Source: CAD feature listing. Evaluate the final solid. Frame: model axes, mm. A direction names the side the tool comes from. Give positions to 0.01 mm unless a question says otherwise; leave off trailing zeros. Order: outer loops, then holes, each group sorted by start corner. A loop starts at its lowest first (then second) coordinate and runs counter-clockwise, first axis right, second up.
from build123d import *

# Parameters (mm, degrees)
BOSS_EXTRUDE1_DEPTH = 120
BOSS_EXTRUDE2_DEPTH = 120
SKETCH4_W           = 0.8
SKETCH4_H           = 47.4
BOSS_EXTRUDE3_DEPTH = 120
BOSS_EXTRUDE4_DEPTH = 6
SKETCH6_W           = 3.197214061
SKETCH6_H           = 10
SKETCH6_W_2         = 2.544721395
CUT_EXTRUDE1_DEPTH  = 90
SKETCH7_W           = 91.376615624
SKETCH7_H           = 120.194280457
CUT_EXTRUDE3_DEPTH  = 258
SKETCH8_W           = 8
SKETCH8_H           = 30.385133663
CUT_EXTRUDE4_DEPTH  = 4
SKETCH9_R           = 1.35
CUT_EXTRUDE5_DEPTH  = 11
SKETCH10_W          = 29
SKETCH10_H          = 3.5
CUT_EXTRUDE6_DEPTH  = 10
SKETCH11_W          = 115.146040633
SKETCH11_H          = 26.021704098
CUT_EXTRUDE7_DEPTH  = 103
SKETCH12_W          = 27.624810525
SKETCH12_H          = 10
CUT_EXTRUDE8_DEPTH  = 2.5
SKETCH13_R          = 1.35
CUT_EXTRUDE9_DEPTH  = 5


with BuildPart() as part:
    # Sketch1 → Boss-Extrude1 (new body)
    with BuildSketch(Plane(origin=(0, 0, 0), x_dir=(1, 0, 0), z_dir=(0, 1, 0))):
        with BuildLine():
            Line((-55.813088795, 29.403372847), (-55.813088795, -22.596627153))
            ThreePointArc((-55.813088795, -22.596627153), (-52.766075655, -30.195969229), (-45.313088795, -33.585257641))
            Line((-45.313088795, -33.585257641), (-45.313088795, -31.296627153))
            ThreePointArc((-45.313088795, -31.296627153), (-50.969943044, -28.953481402), (-53.313088795, -23.296627153))
            Line((-53.313088795, -23.296627153), (-53.313088795, 30.103372847))
            ThreePointArc((-53.313088795, 30.103372847), (-50.969943044, 35.760227097), (-45.313088795, 38.103372847))
            Line((-45.313088795, 38.103372847), (-45.313088795, 40.392003335))
            ThreePointArc((-45.313088795, 40.392003335), (-52.766075655, 37.002714924), (-55.813088795, 29.403372847))
        make_face()
        with BuildLine():
            Line((-45.313088795, -31.296627153), (-45.313088795, -33.585257641))
            ThreePointArc((-45.313088795, -33.585257641), (-45.063153419, -33.593784407), (-44.813088795, -33.596627153))
            Line((-44.813088795, -33.596627153), (7.186911205, -33.596627153))
            ThreePointArc((7.186911205, -33.596627153), (14.965085798, -30.374801746), (18.186911205, -22.596627153))
            Line((18.186911205, -22.596627153), (18.186911205, 29.403372847))
            ThreePointArc((18.186911205, 29.403372847), (14.965085798, 37.18154744), (7.186911205, 40.403372847))
            Line((7.186911205, 40.403372847), (-45.313088795, 40.403372847))
            Line((-45.313088795, 40.403372847), (-45.313088795, 40.392003335))
            Line((-45.313088795, 40.392003335), (-45.313088795, 38.103372847))
            Line((-45.313088795, 38.103372847), (7.686911205, 38.103372847))
            ThreePointArc((7.686911205, 38.103372847), (13.343765455, 35.760227097), (15.686911205, 30.103372847))
            Line((15.686911205, 30.103372847), (15.686911205, -23.296627153))
            ThreePointArc((15.686911205, -23.296627153), (13.343765455, -28.953481402), (7.686911205, -31.296627153))
            Line((7.686911205, -31.296627153), (-45.313088795, -31.296627153))
        make_face()
    extrude(amount=BOSS_EXTRUDE1_DEPTH)

    # Sketch3 → Boss-Extrude2 (add)
    with BuildSketch(Plane.XZ):
        Polygon((-49.013088795, 31.972735522), (-49.013088795, -37.623215713), (-53.336517426, -34.913867104), (-55.11106611, -29.984565206), (-55.11106611, -26.811210851), (-55.11106611, 25.452378342), (-53.652842224, 27.779331351), (-52.073193111, 30.226675048), align=None)
        Polygon((11.386911205, 31.972735522), (11.386911205, -38.487790626), (13.269736219, -37.809973621), (16.737085445, -32.276969537), (16.568342629, -31.170966754), (16.568342629, 24.789777041), (15.03852436, 28.997230807), align=None)
    extrude(amount=-BOSS_EXTRUDE2_DEPTH)

    # Sketch4 → Boss-Extrude3 (add)
    with BuildSketch(Plane.XZ):
        with Locations((10.986911205, -3.403372847)):
            Rectangle(SKETCH4_W, SKETCH4_H)
        with Locations((-48.613088795, -3.403372847)):
            Rectangle(SKETCH4_W, SKETCH4_H)
    extrude(amount=-BOSS_EXTRUDE3_DEPTH)

    # Sketch5 → Boss-Extrude4 (add)
    with BuildSketch(Plane.XZ):
        with BuildLine():
            ThreePointArc((-49.013088795, 30.389581403), (-52.154141346, 27.443915423), (-53.313088795, 23.296627153))
            Line((-53.313088795, 23.296627153), (-53.313088795, -30.103372847))
            ThreePointArc((-53.313088795, -30.103372847), (-52.154141346, -34.250661118), (-49.013088795, -37.196327098))
            Line((-49.013088795, -37.196327098), (-49.013088795, -27.103372847))
            Line((-49.013088795, -27.103372847), (-48.213088795, -27.103372847))
            Line((-48.213088795, -27.103372847), (-48.213088795, 20.296627153))
            Line((-48.213088795, 20.296627153), (-49.013088795, 20.296627153))
            Line((-49.013088795, 20.296627153), (-49.013088795, 30.389581403))
        make_face()
        with BuildLine():
            ThreePointArc((11.386911205, -37.196327098), (14.527963756, -34.250661118), (15.686911205, -30.103372847))
            Line((15.686911205, -30.103372847), (15.686911205, 23.296627153))
            ThreePointArc((15.686911205, 23.296627153), (14.527963756, 27.443915423), (11.386911205, 30.389581403))
            Line((11.386911205, 30.389581403), (11.386911205, 20.296627153))
            Line((11.386911205, 20.296627153), (10.586911205, 20.296627153))
            Line((10.586911205, 20.296627153), (10.586911205, -27.103372847))
            Line((10.586911205, -27.103372847), (11.386911205, -27.103372847))
            Line((11.386911205, -27.103372847), (11.386911205, -37.196327098))
        make_face()
    extrude(amount=BOSS_EXTRUDE4_DEPTH)

    # Sketch6 → Cut-Extrude1 (cut)
    with BuildSketch(Plane.XZ.offset(6)):
        with Locations((-49.114481764, 12.296627153)):
            Rectangle(SKETCH6_W, SKETCH6_H)
        with Locations((-49.440728097, -19.103372847)):
            Rectangle(SKETCH6_W_2, SKETCH6_H)
        with Locations((11.814550508, -19.103372847)):
            Rectangle(SKETCH6_W_2, SKETCH6_H)
        with Locations((11.488304175, 12.296627153)):
            Rectangle(SKETCH6_W, SKETCH6_H)
    extrude(amount=-CUT_EXTRUDE1_DEPTH, mode=Mode.SUBTRACT)

    # Sketch7 → Cut-Extrude3 (cut)
    with BuildSketch(Plane.XZ.offset(6)):
        with Locations((0.375219017, -9.755963426)):
            Rectangle(SKETCH7_W, SKETCH7_H)
    extrude(amount=-CUT_EXTRUDE3_DEPTH, mode=Mode.SUBTRACT)

    # Sketch8 → Cut-Extrude4 (cut)
    with BuildSketch(Plane(origin=(-48.213088795, 0, 0), x_dir=(0, 0, -1), z_dir=(1, 0, 0))):
        with Locations((3.403372847, 3.807433168)):
            Rectangle(SKETCH8_W, SKETCH8_H)
    extrude(amount=-CUT_EXTRUDE4_DEPTH, mode=Mode.SUBTRACT)

    # Sketch9 → Cut-Extrude5 (cut)
    with BuildSketch(Plane(origin=(-48.213088795, 0, 0), x_dir=(0, 0, -1), z_dir=(1, 0, 0))):
        with Locations((-3.969366177, -3)):
            Circle(SKETCH9_R)
        with Locations((10.753372847, -3)):
            Circle(SKETCH9_R)
        with Locations((-20.319366177, -3)):
            Circle(SKETCH9_R)
        with Locations((27.103372847, -3)):
            Circle(SKETCH9_R)
    extrude(amount=-CUT_EXTRUDE5_DEPTH, mode=Mode.SUBTRACT)

    # Sketch10 → Cut-Extrude6 (cut)
    with BuildSketch(Plane.ZY.offset(55.813088795)):
        with Locations((-3.403372847, 97.75)):
            Rectangle(SKETCH10_W, SKETCH10_H)
    extrude(amount=-CUT_EXTRUDE6_DEPTH, mode=Mode.SUBTRACT)

    # Sketch11 → Cut-Extrude7 (cut)
    with BuildSketch(Plane.ZY.offset(55.813088795)):
        with Locations((0.013322813, 115.510852049)):
            Rectangle(SKETCH11_W, SKETCH11_H)
    extrude(amount=-CUT_EXTRUDE7_DEPTH, mode=Mode.SUBTRACT)

    # Sketch12 → Cut-Extrude8 (cut)
    with BuildSketch(Plane(origin=(-48.213088795, 0, 0), x_dir=(0, 0, -1), z_dir=(1, 0, 0))):
        with Locations((4.217176257, 79)):
            Rectangle(SKETCH12_W, SKETCH12_H)
    extrude(amount=-CUT_EXTRUDE8_DEPTH, mode=Mode.SUBTRACT)

    # Sketch13 → Cut-Extrude9 (cut)
    with BuildSketch(Plane.ZY.offset(55.813088795)):
        with Locations((-23.403372847, 98.5)):
            Circle(SKETCH13_R)
        with Locations((16.596627153, 98.5)):
            Circle(SKETCH13_R)
    extrude(amount=-CUT_EXTRUDE9_DEPTH, mode=Mode.SUBTRACT)


solid = part.part
1) Section query A-A on z = 9. Output: boundary loops of the cut face in (x, y).
Checks:
outline: (-55.81, 0) - (-53.31, 0) - (-53.31, -6) - (-50.71, -6) - (-50.71, 84) - (-48.21, 84) - (-48.21, 96) - (-55.81, 96) - close; (-55.81, 99.5) - (-48.21, 99.5) - (-48.21, 102.5) - (-55.81, 102.5) - close
2) Section query C-C on y = 52.5. Output: boundary loops of the cut face in (x, z).
Checks:
outline: (-55.81, -29.4) arc R11 ccw to (-45.31, -40.39) - (-45.31, -38.1) arc R8 cw to (-49.01, -37.2) - (-49.01, -27.1) - (-48.21, -27.1) - (-48.21, -24.1) - (-50.71, -24.1) - (-50.71, -14.1) - (-48.21, -14.1) - (-48.21, 7.3) - (-50.71, 7.3) - (-50.71, 17.3) - (-48.21, 17.3) - (-48.21, 20.3) - (-49.01, 20.3) - (-49.01, 30.39) arc R8 cw to (-45.31, 31.3) - (-45.31, 33.59) arc R11 ccw to (-55.81, 22.6) - close
3) Section query B-B on y = -3. State how many separate pieces and enclosed holes the cut face has, and give its area (3 significant figures).
Checks:
separate pieces: 5
enclosed holes: 0
area: 176 mm2
4) Reachability of faces 5 (the face through (-50.813, 99, 17)), 6 (the face through (-50, 6, 0.597)), 7 (the face through (-49.013, 49, 25)) from +Z, -Z, +X, -X, +Y, -Y: full face, straight path, thin tool, end or side. Return the list, or none.
Checks:
face 5: -X
face 6: +X, -Y
face 7: +X, +Y, -Y
5) Pull-direction query (Z, two-part tool) for faces 1 (the face through (-53.348, 97.302, -22.78)), 2 (the face through (-50, 6, -7.403)), 3 (the face through (-52.12, -2.96, 27.5)), 4 (the face through (-53.313, -3, -3)); classes: +Z half, -Z half, draft (parallel to the pull), parting line (faces both ways), or undercut.
Checks:
face 1: undercut
face 2: undercut
face 3: +Z half
face 4: draft
6) First-contact query: pin 1 Ø2.5 at (y, z) = (-3, -10.75) entering from -X; pin 2 Ø1.2 at (x, y) = (-49.5, 15) entering from +Z; pin 3 Ø12 at (y, z) = (16.5, 17.5) entering from +X; pin 4 Ø6 at (x, y) = (-53, 20.5) entering from +Z. Flat tips, straight axial feed; report the tip coordinate or a pass-through.
Checks:
pin 1: passes through
pin 2: stops at z = 32.81
pin 3: stops at x = -48.21
pin 4: stops at z = 32.3
7) Section query D-D on z = -35. Output: boundary loops of the cut face in (x, y).
Checks:
outline: (-54.28, 0) - (-51.64, 0) - (-51.64, -6) - (-49.01, -6) - (-49.01, 102.5) - (-54.28, 102.5) - close
8) Ray query, L1, parallel to Y at x = -48.75, z = 1; L2, parallel to Y at x = -55.5, z = 6; L3, parallel to Y at x = -50.25, z = 10.5. Return the intervals inside material, ascending.
Checks:
L1: y = -6 to 74, 84 to 96, 99.5 to 102.5
L2: y = 0 to 96, 99.5 to 102.5
L3: y = 84 to 96, 99.5 to 102.5
